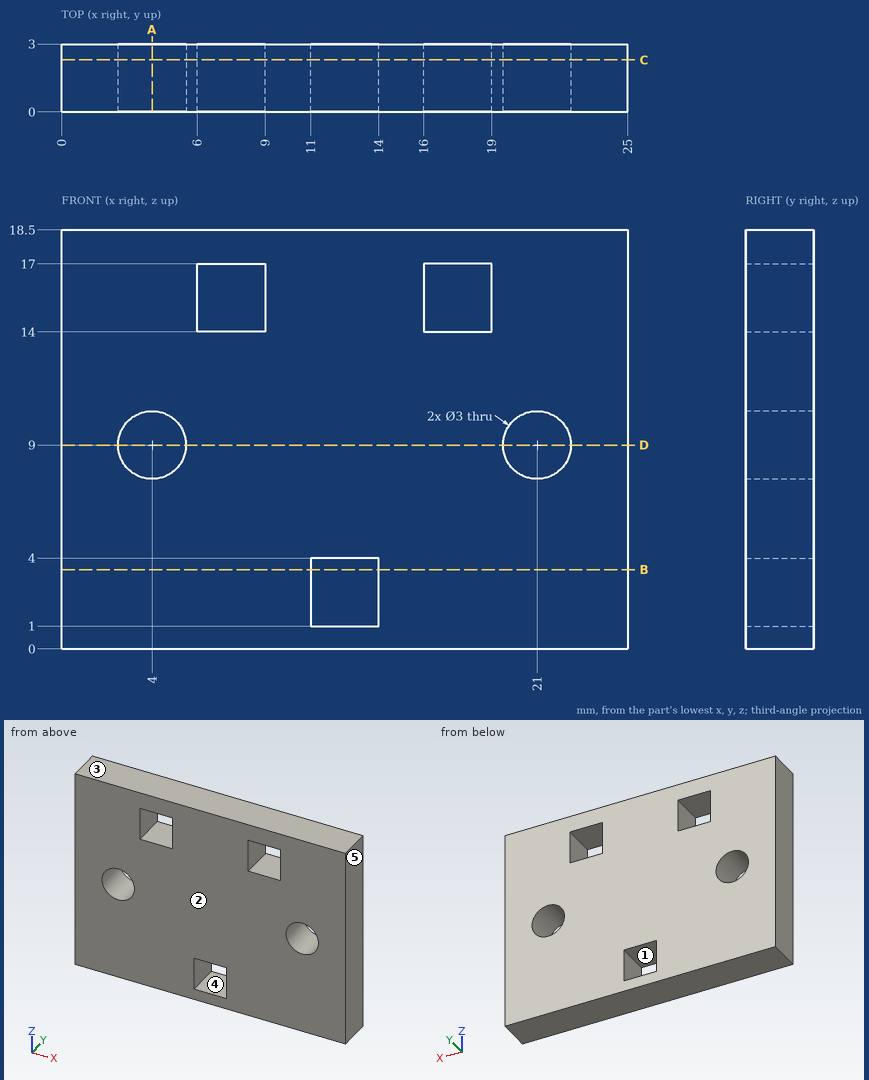
Drawing for the job (mm, zero at the part's lowest x, y, z). A direction names the side the tool comes from. Give positions to 0.01 mm unless a question says otherwise; leave off trailing zeros. Order: outer loops, then holes, each group sorted by start corner. A loop starts at its lowest first (then second) coordinate and runs counter-clockwise, first axis right, second up. Notation, with made-up numbers: (43.25, 70.5) -> (48.25, 70.5) arc R15 ccw to (48.25, 91.5) -> close; hole circle Ø3 at (3.5, 52). An arc over 180 degrees is marked (long way). Use one line per item in the form item = value.
(1) Tool access for the marked faces 1 and 2: list every direction of +Z, -Z, +X, -X, +Y, -Y with a clear straight run to the whole face (end or side of a thin tool).
Solution:
face_1 = +Y, -Y
face_2 = +Z, -Z, +X, -X, -Y
(2) Saw through at D-D (z = 9). Write the cut outline in (x, y).
Solution:
outline = (0, 0) -> (2.5, 0) -> (2.5, 3) -> (0, 3) -> close; (5.5, 0) -> (19.5, 0) -> (19.5, 3) -> (5.5, 3) -> close; (22.5, 0) -> (25, 0) -> (25, 3) -> (22.5, 3) -> close
(3) Saw through at B-B (z = 3.5). Write the cut outline in (x, y).
Solution:
outline = (0, 0) -> (11, 0) -> (11, 3) -> (0, 3) -> close; (14, 0) -> (25, 0) -> (25, 3) -> (14, 3) -> close
(4) Saw through at C-C (y = 2.3). Write the cut outline in (x, z).
Solution:
outline = (0, 0) -> (25, 0) -> (25, 18.5) -> (0, 18.5) -> close; hole circle Ø3 at (4, 9); hole (6, 14) -> (9, 14) -> (9, 17) -> (6, 17) -> close; hole (11, 1) -> (14, 1) -> (14, 4) -> (11, 4) -> close; hole (16, 14) -> (19, 14) -> (19, 17) -> (16, 17) -> close; hole circle Ø3 at (21, 9)
(5) Flat gauge pins, fed straight in: P1, Ø0.9, axis at y = 1, z = 15, coming from the -X side; P2, Ø2.5, axis at x = 21, z = 9, coming from the +Y side. Where does each tip first touch, or does it go through?
Solution:
P1 = 0
P2 = through
(6) Drill centre lines: line 1 (X direction, y = 1.6, z = 14.25); line 2 (Z direction, x = 4, y = 0.7); line 3 (Z direction, x = 13.5, y = 1.05). Where is each one in solid material? Low to high. Write a range as from..to.
Solution:
line_1 = 0..6, 9..16, 19..25
line_2 = 0..7.5, 10.5..18.5
line_3 = 0..1, 4..18.5
(7) Pull direction Z, two halves, no side cores. Call the marked faces 3, 4 and 5: +Z half, -Z half, draft (parallel to the pull), parting line (faces both ways), or undercut.
Solution:
face_3 = +Z half
face_4 = undercut
face_5 = draft
(8) Saw through at A-A (x = 4). Write the cut outline in (y, z).
Solution:
outline = (0, 0) -> (3, 0) -> (3, 7.5) -> (0, 7.5) -> close; (0, 10.5) -> (3, 10.5) -> (3, 18.5) -> (0, 18.5) -> close
